Can you work these out from the model? Positions are in its coordinate system, mm. Face numbers are marked on the shaded views. A direction names the side the tool comes from. Round coordinates to 2 decimals unless told otherwise and drop trailing zeros. Order: outer loops, then holes, each group sorted by start corner. A loop starts at its lowest first (then second) coordinate and runs counter-clockwise, first axis right, second up. Notation, with made-up numbers: (56.5, 29.5) - (64.5, 29.5) arc R18 cw to (64.5, 33.5) - close; hole circle Ø2 at (25, 48.5). An arc over 180 degrees is marked (long way). Write item = value, one per line.
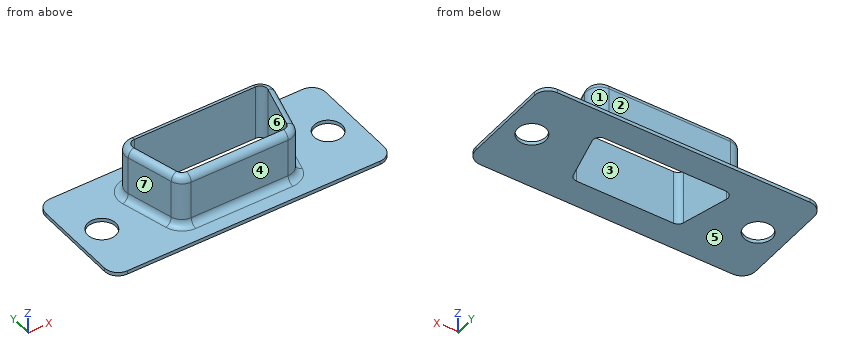
from build123d import *

# Parameters (mm, degrees)
SKETCH1_R           = 1.55
BOSS_EXTRUDE1_DEPTH = 0.4
BOSS_EXTRUDE2_DEPTH = 5.7
FILLET1_R           = 0.75


with BuildPart() as part:
    # Sketch1 → Boss-Extrude1 (new body)
    with BuildSketch(Plane.XY):
        with BuildLine():
            Line((-13.95, 6.25), (13.95, 6.25))
            ThreePointArc((13.95, 6.25), (15.010660172, 5.810660172), (15.45, 4.75))
            Line((15.45, 4.75), (15.45, -4.75))
            ThreePointArc((15.45, -4.75), (15.010660172, -5.810660172), (13.95, -6.25))
            Line((13.95, -6.25), (-13.95, -6.25))
            ThreePointArc((-13.95, -6.25), (-15.010660172, -5.810660172), (-15.45, -4.75))
            Line((-15.45, -4.75), (-15.45, 4.75))
            ThreePointArc((-15.45, 4.75), (-15.010660172, 5.810660172), (-13.95, 6.25))
        make_face()
        with Locations((-12.5, 0)):
            Circle(SKETCH1_R, mode=Mode.SUBTRACT)
        with Locations((12.5, 0)):
            Circle(SKETCH1_R, mode=Mode.SUBTRACT)
        with BuildLine():
            Line((-6.697085729, 3.25), (6.697085729, 3.25))
            ThreePointArc((6.697085729, 3.25), (7.292100735, 2.956571072), (7.421530099, 2.305885716))
            Line((7.421530099, 2.305885716), (6.081784137, -2.694114284))
            ThreePointArc((6.081784137, -2.694114284), (5.813910839, -3.095015005), (5.357339767, -3.25))
            Line((5.357339767, -3.25), (-5.357339767, -3.25))
            ThreePointArc((-5.357339767, -3.25), (-5.813910839, -3.095015005), (-6.081784137, -2.694114284))
            Line((-6.081784137, -2.694114284), (-7.421530099, 2.305885716))
            ThreePointArc((-7.421530099, 2.305885716), (-7.292100735, 2.956571072), (-6.697085729, 3.25))
        make_face(mode=Mode.SUBTRACT)
    extrude(amount=BOSS_EXTRUDE1_DEPTH)

    # Sketch2 → Boss-Extrude2 (add)
    with BuildSketch(Plane.XY.offset(0.4)):
        with BuildLine():
            Line((6.697085729, 4), (-6.697085729, 4))
            ThreePointArc((-6.697085729, 4), (-7.88711574, 3.413142144), (-8.145974469, 2.111771432))
            Line((-8.145974469, 2.111771432), (-6.806228507, -2.888228568))
            ThreePointArc((-6.806228507, -2.888228568), (-6.270481911, -3.69003001), (-5.357339767, -4))
            Line((-5.357339767, -4), (5.357339767, -4))
            ThreePointArc((5.357339767, -4), (6.270481911, -3.69003001), (6.806228507, -2.888228568))
            Line((6.806228507, -2.888228568), (8.145974469, 2.111771432))
            ThreePointArc((8.145974469, 2.111771432), (7.88711574, 3.413142144), (6.697085729, 4))
        make_face()
        with BuildLine():
            Line((-7.421530099, 2.305885716), (-6.081784137, -2.694114284))
            ThreePointArc((-6.081784137, -2.694114284), (-5.813910839, -3.095015005), (-5.357339767, -3.25))
            Line((-5.357339767, -3.25), (5.357339767, -3.25))
            ThreePointArc((5.357339767, -3.25), (5.813910839, -3.095015005), (6.081784137, -2.694114284))
            Line((6.081784137, -2.694114284), (7.421530099, 2.305885716))
            ThreePointArc((7.421530099, 2.305885716), (7.292100735, 2.956571072), (6.697085729, 3.25))
            Line((6.697085729, 3.25), (-6.697085729, 3.25))
            ThreePointArc((-6.697085729, 3.25), (-7.292100735, 2.956571072), (-7.421530099, 2.305885716))
        make_face(mode=Mode.SUBTRACT)
    extrude(amount=BOSS_EXTRUDE2_DEPTH)

    # Fillet1
    fillet1_edges = [part.edges().sort_by_distance(p)[0] for p in [
        (-6.270481911, -3.69003001, 6.1),
        (0, -4, 6.1),
        (6.270481911, -3.69003001, 6.1),
        (7.476101488, -0.388228568, 6.1),
        (7.88711574, 3.413142144, 6.1),
        (0, 4, 6.1),
        (-7.88711574, 3.413142144, 6.1),
        (-7.476101488, -0.388228568, 6.1),
        (-6.270481911, -3.69003001, 0.4),
        (0, -4, 0.4),
        (6.270481911, -3.69003001, 0.4),
        (7.476101488, -0.388228568, 0.4),
        (7.88711574, 3.413142144, 0.4),
        (0, 4, 0.4),
        (-7.88711574, 3.413142144, 0.4),
        (-7.476101488, -0.388228568, 0.4),
    ]]
    fillet(fillet1_edges, radius=FILLET1_R - 0.0001)  # a hair under: the kernel refuses the full size


solid = part.part
(1) On a 3-axis mill with a long thin cutter (end or side, diameter ignored), from which of +Z, -Z, +X, -X, +Y, -Y can I reach the whole of each face in a straight line? I mean the marked faces 4, 5, 6 and 7. Say none if no direction works.
Computed:
face_4 = +Z, +X, -X, -Y
face_5 = -Z, +X, -X, +Y, -Y
face_6 = +Z, -Z
face_7 = +Z, -X, -Y
(2) If I drill on line 1 (Y direction, x = 12.5, z = 0.15); line 2 (Y direction, x = 3.5, z = 5); line 3 (X direction, y = 1.25, z = 0.75), over which ranges is the centre line in solid material (lowest first)? Write a range as from..to.
Computed:
line_1 = -6.25..-1.55, 1.55..6.25
line_2 = -4..-3.25, 3.25..4
line_3 = -8.03..-7.14, 7.14..8.03
(3) If we section it at B-B (z = 4.75): Write out the boundary of the cut face in (x, y).
Computed:
outline = (-8.15, 2.11) - (-6.81, -2.89) arc R1.5 ccw to (-5.36, -4) - (5.36, -4) arc R1.5 ccw to (6.81, -2.89) - (8.15, 2.11) arc R1.5 ccw to (6.7, 4) - (-6.7, 4) arc R1.5 ccw to start; hole (-7.42, 2.31) - (-6.08, -2.69) arc R0.75 ccw to (-5.36, -3.25) - (5.36, -3.25) arc R0.75 ccw to (6.08, -2.69) - (7.42, 2.31) arc R0.75 ccw to (6.7, 3.25) - (-6.7, 3.25) arc R0.75 ccw to start
(4) Will these pins go through, and if not, where does the flat tip stop? P1, Ø3, axis at x = 1.5, z = 3, coming from the +Y side; P2, Ø3, axis at x = 0, z = 2.5, coming from the -Y side; P3, Ø2, axis at y = -3.5, z = 5, coming from the -X side.
Computed:
P1 = 4
P2 = -4.02
P3 = -6.91
(5) Thinking about a two-plate mould opening in X: for the marked faces 1, 2 and 3, which applies, +X half, -X half, draft (parallel to the pull), parting line (faces both ways), or undercut?
Computed:
face_1 = +X half
face_2 = draft
face_3 = undercut
(6) If we section it at A-A (x = 12.5): Write out the boundary of the cut face in (y, z), plus the area to 3 significant figures.
Computed:
outline = (-6.25, 0) - (-1.55, 0) - (-1.55, 0.4) - (-6.25, 0.4) - close; (1.55, 0) - (6.25, 0) - (6.25, 0.4) - (1.55, 0.4) - close
area = 3.76 mm^2
